Design review of the part built by this model. Coordinates are the model's own, in mm. Face numbers are marked on the shaded views. Give positions to 0.01 mm unless a question says otherwise; leave off trailing zeros. Loops run counter-clockwise (first coordinate to the right, second up) from the corner with the lowest first, then second, coordinate; pieces in that order, holes last.
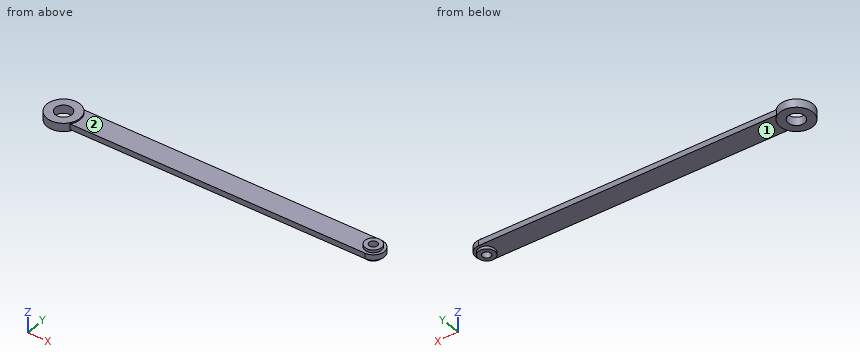
from build123d import *

# Parameters (mm, degrees)
SKETCH2_R                = 6000
SKETCH2_R_2              = 3000
BOSS_EXTRUDE1_DEPTH      = 3000
BOSS_EXTRUDE2_DEPTH      = 1000
BOSS_EXTRUDE2_DEPTH_BACK = 1000
BOSS_EXTRUDE3_DEPTH      = 1000
BOSS_EXTRUDE3_DEPTH_BACK = 3000
SKETCH4_R                = 3000
SKETCH5_R                = 1500
CUT_EXTRUDE1_DEPTH       = 5000
SCALE1_SCALE             = 0.001


with BuildPart() as part:
    # Sketch2 → Boss-Extrude1 (new body)
    with BuildSketch(Plane.XY):
        Circle(SKETCH2_R)
        Circle(SKETCH2_R_2, mode=Mode.SUBTRACT)
    extrude(amount=BOSS_EXTRUDE1_DEPTH)

    # Sketch3 → Boss-Extrude2 (add, two sides: drawn at the far end of the back side and taken through both)
    with BuildSketch(Plane.XY.offset(1500).offset(-BOSS_EXTRUDE2_DEPTH_BACK)):
        with BuildLine():
            Line((1140.414956358, 4594.307428083), (112000, 4594.307428083))
            ThreePointArc((112000, 4594.307428083), (116000, 594.307428083), (112000, -3405.692571917))
            Line((112000, -3405.692571917), (3287.775102105, -3405.692571917))
            ThreePointArc((3287.775102105, -3405.692571917), (4571.894224331, 1227.187930987), (1140.414956358, 4594.307428083))
        make_face()
    extrude(amount=BOSS_EXTRUDE2_DEPTH + BOSS_EXTRUDE2_DEPTH_BACK)

    # Sketch4 → Boss-Extrude3 (add, two sides: drawn at the far end of the back side and taken through both)
    with BuildSketch(Plane(origin=(0, 0, 500), x_dir=(-1, 0, 0), z_dir=(0, 0, -1)).offset(-BOSS_EXTRUDE3_DEPTH_BACK)):
        with Locations((-112000, 594.307428083)):
            Circle(SKETCH4_R)
    extrude(amount=BOSS_EXTRUDE3_DEPTH + BOSS_EXTRUDE3_DEPTH_BACK)

    # Sketch5 → Cut-Extrude1 (cut)
    with BuildSketch(Plane(origin=(0, 0, -500), x_dir=(-1, 0, 0), z_dir=(0, 0, -1))):
        with Locations((-112000, 594.307428083)):
            Circle(SKETCH5_R)
    extrude(amount=-CUT_EXTRUDE1_DEPTH, mode=Mode.SUBTRACT)


with BuildPart() as part_1:
    # Scale1: scaled about (53497.162872558, 525.016851584, 1500)
    add(part.part.scale(SCALE1_SCALE).moved(Location((53443.665709685, 524.491834732, 1498.5))))


solid = part_1.part
Q1. Take a section at B-B (x = 53510.5). Give the boundary of the cut face in (y, z), plus the area to 3 significant figures.
Results:
outline: (521.09, 1499) - (529.09, 1499) - (529.09, 1501) - (521.09, 1501) - close
area: 16.0 mm2
Q2. Draft analysis for pull direction X (two halves, no side actions). For the marked faces 1 and 2, state which applies: pulls with the +X half, pulls with the -X half, needs draft (parallel to the pull), parting line crosses it, or undercut.
Results:
face 1: undercut
face 2: undercut
Q3. Wall thickness on line 1 (Z direction, x = 53503, y = 524.75); line 2 (Y direction, x = 53505, z = 1500.9); line 3 (X direction, y = 524.25, z = 1499.8): over which ranges is each line inside the solid? List them lowest first.
Results:
line 1: z = 1499 to 1501
line 2: y = 521.09 to 529.09
line 3: x = 53437.67 to 53440.68, 53446.66 to 53554.42, 53556.91 to 53559.58
Q4. Insertion check: pin 1 (5 mm diameter, centred on x = 53471.5, y = 521.5, fed in from -Z); pin 2 (0.6 mm diameter, centred on x = 53481.5, z = 1499.5, fed in from +Y); pin 3 (6 mm diameter, centred on x = 53444, y = 527, fed in from -Z). Each pin has a flat end and moves straight along its axis. Give the tip position at first contact, or say it passes through.
Results:
pin 1: stops at z = 1499
pin 2: stops at y = 529.09
pin 3: stops at z = 1498.5
Q5. Take a section at A-A (z = 1500.25). Give the boundary of the cut face in (x, y), plus the area to 3 significant figures.
Results:
outline: (53447.52, 529.09) arc R6 ccw (long way) to (53448.61, 521.09) - (53555.67, 521.09) arc R4 ccw to (53555.67, 529.09) - close; hole circle Ø6 at (53443.67, 524.49); hole circle Ø3 at (53555.67, 525.09)
area: 955 mm2
